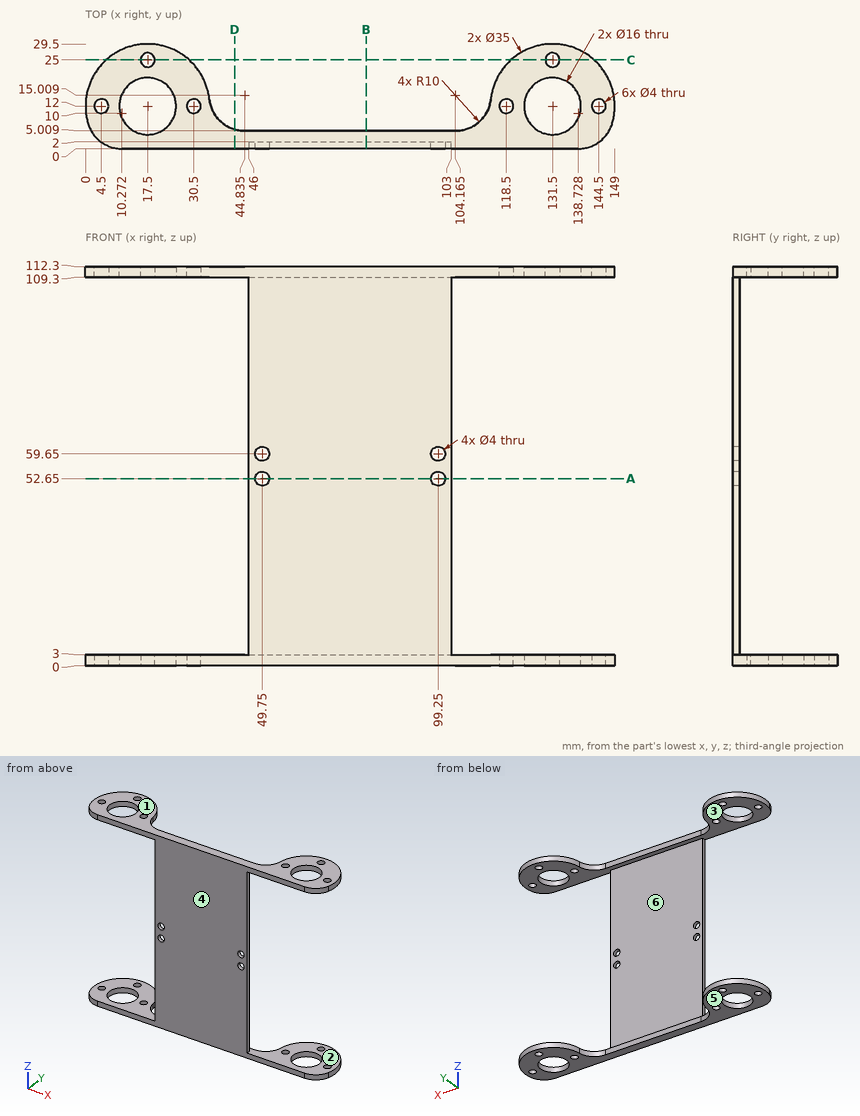
Answer from the drawing. Dimensions are ordinates in mm from the lowest x, y and z of the part. A direction names the side the tool comes from. Give positions to 0.01 mm unless a question says otherwise; leave off trailing zeros. Write each loop counter-clockwise with the first axis right and the second up, starting at its lowest first coordinate (ties: lowest second). Pieces come first, ordered by that corner, then holes.
1) Section C-C (y = 25) is taken. Count the separate pieces of the cut face and the enclosed holes in it, and give its area (3 significant figures).
2) Find the intervals of material crossed by L1, parallel to Z at x = 99.5, y = 1.5 (1 decimal); L2, parallel to Z at x = 138.5, y = 17.5; L3, parallel to Y at x = 49, z = 102, in increasing order.
3) A tool of negligible diameter and unlimited length cuts with its end or side. For the marked faces 5 and 6, from which of +Z, -Z, +X, -X, +Y, -Y can it reach the whole face along a straight path? Write none if from no direction.
4) Section A-A (z = 52.65) is taken. Write down the section's boundary in (x, y).
5) For a pull along Z with two mould halves and no side action, classify the marked faces 1, 2, 3 and 4 as pulls with the +Z half, pulls with the -Z half, needs draft (parallel to the pull), parting line crosses it, or undercut.
6) Given P1, Ø5, axis at x = 55.5, z = 30.5, coming from the +Y side; P2, Ø1.5, axis at x = 81, z = 110, coming from the +Y side, each flat-ended and moving along its own axis, determine where each tip first touches the part or whether it passes through.
7) Section B-B (x = 79) is taken. Write down the section's boundary in (y, z).
8) Section D-D (x = 42) is taken. Write down the section's boundary in (y, z), and give its area (3 significant figures).
Response:
1. separate pieces: 8
1. enclosed holes: 0
1. area: 233 mm2
2. L1: z = 0 to 50.7, 54.6 to 57.7, 61.6 to 112.3
2. L2: z = 0 to 3, 109.3 to 112.3
2. L3: y = 0 to 2
3. face 5: -Z, +X, -X, +Y, -Y
3. face 6: +X, -X, +Y
4. outline: (46, 0) - (47.75, 0) - (47.75, 2) - (46, 2) - close; (51.75, 0) - (97.25, 0) - (97.25, 2) - (51.75, 2) - close; (101.25, 0) - (103, 0) - (103, 2) - (101.25, 2) - close
5. face 1: pulls with the +Z half
5. face 2: undercut
5. face 3: undercut
5. face 4: needs draft
6. P1: stops at y = 2
6. P2: stops at y = 5.01
7. outline: (0, 0) - (5.01, 0) - (5.01, 3) - (2, 3) - (2, 109.3) - (5.01, 109.3) - (5.01, 112.3) - (0, 112.3) - close
8. outline: (0, 0) - (5.42, 0) - (5.42, 3) - (0, 3) - close; (0, 109.3) - (5.42, 109.3) - (5.42, 112.3) - (0, 112.3) - close
8. area: 32.5 mm2
